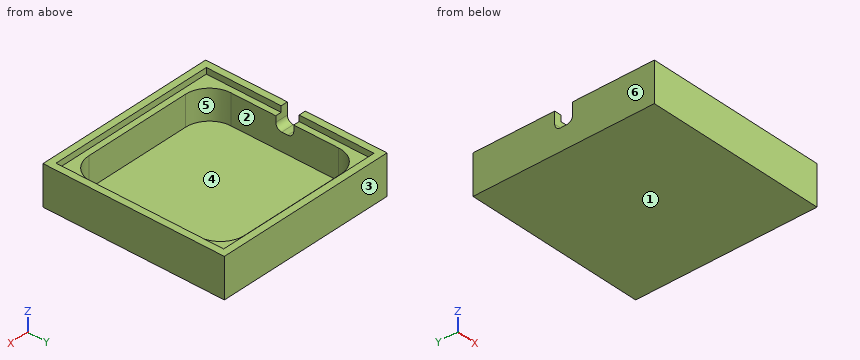
```python
from build123d import *

# Parameters (mm, degrees)
SKETCH_W      = 30.3
SKETCH_H      = 30.3
PAD_DEPTH     = 0.6
SKETCH001_W   = 28
SKETCH001_H   = 28
PAD001_DEPTH  = 5
SKETCH003_W   = 30.3
SKETCH003_H   = 30.3
SKETCH003_W_2 = 28
SKETCH003_H_2 = 28
PAD002_DEPTH  = 6
POCKET_DEPTH  = 2.15


with BuildPart() as part:
    # Sketch → Pad (new body)
    with BuildSketch(Plane.XY):
        Rectangle(SKETCH_W, SKETCH_H)
    extrude(amount=PAD_DEPTH)

    # Sketch001 (on Face6 of Pad) → Pad001 (join)
    with BuildSketch(Plane.XY.offset(0.6)):
        Rectangle(SKETCH001_W, SKETCH001_H)
        with BuildLine():
            Line((-9, 13), (9, 13))
            ThreePointArc((13, 9), (11.828427, 11.828427), (9, 13))
            Line((13, 9), (13, -9))
            ThreePointArc((9, -13), (11.828427, -11.828427), (13, -9))
            Line((9, -13), (-9, -13))
            ThreePointArc((-13, -9), (-11.828427, -11.828427), (-9, -13))
            Line((-13, -9), (-13, 9))
            ThreePointArc((-9, 13), (-11.828427, 11.828427), (-13, 9))
        make_face(mode=Mode.SUBTRACT)
    extrude(amount=PAD001_DEPTH)

    # Sketch003 (on Face5 of Pad001) → Pad002 (join)
    with BuildSketch(Plane.XY.offset(0.6)):
        Rectangle(SKETCH003_W, SKETCH003_H)
        Rectangle(SKETCH003_W_2, SKETCH003_H_2, mode=Mode.SUBTRACT)
    extrude(amount=PAD002_DEPTH)

    # Sketch004 (on Face7 of Pad002) → Pocket (cut)
    with BuildSketch(Plane(origin=(-15.15, 0, 0), x_dir=(0, -1, 0), z_dir=(-1, 0, 0))):
        with BuildLine():
            Line((-1.5, 6.6), (1.5, 6.6))
            Line((1.5, 6.6), (1.5, 4.6))
            ThreePointArc((0.5, 3.6), (1.207107, 3.892893), (1.5, 4.6))
            Line((0.5, 3.6), (-0.5, 3.6))
            ThreePointArc((-1.5, 4.6), (-1.207107, 3.892893), (-0.5, 3.6))
            Line((-1.5, 4.6), (-1.5, 6.6))
        make_face()
    extrude(amount=-POCKET_DEPTH, mode=Mode.SUBTRACT)


solid = part.part
```
Check sheet for the modelled part. Datum: model origin and axes. Units: mm. Face numbers are marked on the shaded views. A direction names the side the tool comes from. Coordinates: 2 decimals unless noted, no trailing zeros. Write each loop counter-clockwise with the first axis right and the second up, starting at its lowest first coordinate (ties: lowest second). Pieces come first, ordered by that corner, then holes. Notation, with made-up numbers: M 41.5,3.25 L 46.5,3.25 A12 cw 46.5,12.25 Z; hole C -29,81.25 d7. An arc over 180 degrees is marked long. Use one line per item in the form item = value.
Item 1: Sectioned sample at C-C, the plane z = 5. Record the cut outline in (x, y), and give its area (3 significant figures).
Answer below:
outline = M -15.15,-15.15 L 15.15,-15.15 L 15.15,15.15 L -15.15,15.15 L -15.15,1.5 L -13,1.5 L -13,9 A4 cw -9,13 L 9,13 A4 cw 13,9 L 13,-9 A4 cw 9,-13 L -9,-13 A4 cw -13,-9 L -13,-1.5 L -15.15,-1.5 Z
area = 249 mm^2
Item 2: Sectioned sample at B-B, the plane y = 2. Record the cut outline in (x, z), and give its area (3 significant figures).
Answer below:
outline = M -15.15,0 L 15.15,0 L 15.15,6.6 L 14,6.6 L 14,5.6 L 13,5.6 L 13,0.6 L -13,0.6 L -13,5.6 L -14,5.6 L -14,6.6 L -15.15,6.6 Z
area = 42.0 mm^2
Item 3: Gauge pin test, flat ends, axial feed: pin 1 Ø8 at (x, y) = (-2.5, 6) entering from +Z; pin 2 Ø0.8 at (x, y) = (-14.5, 0) entering from +Z. Record the tip position at first contact, or that the pin passes through.
Answer below:
pin_1 = 0.6
pin_2 = 3.6
Item 4: Sectioned sample at A-A, the plane z = 1.75. Record the cut outline in (x, y).
Answer below:
outline = M -15.15,-15.15 L 15.15,-15.15 L 15.15,15.15 L -15.15,15.15 Z; hole M -13,-9 A4 ccw -9,-13 L 9,-13 A4 ccw 13,-9 L 13,9 A4 ccw 9,13 L -9,13 A4 ccw -13,9 Z
Item 5: Release check for a two-part mould opening along Y. For the marked faces 3, 4, 5 and 6 record: pulls with the +Y half, pulls with the -Y half, needs draft (parallel to the pull), parting line crosses it, or undercut.
Answer below:
face_3 = pulls with the +Y half
face_4 = undercut
face_5 = undercut
face_6 = needs draft
Item 6: Set-up check for the marked faces 1 and 2: record each of +Z, -Z, +X, -X, +Y, -Y from which the full face is reachable in a straight line by a thin tool's end or side.
Answer below:
face_1 = -Z, +X, -X, +Y, -Y
face_2 = +Z
Item 7: Material ranges on L1, parallel to X at y = 6.5, z = 5.25; L2, parallel to Y at x = 10, z = 6, recorded low to high. Write a range as from..to.
Answer below:
L1 = -15.15..-13, 13..15.15
L2 = -15.15..-14, 14..15.15
